from build123d import *

# Parameters (mm, degrees)
SKETCH_1_W          = 33
SKETCH_1_H          = 45
EXTRUDE_1_DEPTH     = 17
SKETCH_2_W          = 5
SKETCH_2_H          = 6
CUT_EXTRUDE_1_DEPTH = 44.407948581
SKETCH_4_R          = 3
EXTRUDE_2_DEPTH     = 6


with BuildPart() as part:
    # Эскиз1 → Бобышка-Вытянуть1 (new body)
    with BuildSketch(Plane.XY):
        Rectangle(SKETCH_1_W, SKETCH_1_H)
    extrude(amount=EXTRUDE_1_DEPTH)

    # Эскиз2 → Вырез-Вытянуть1 (cut, through all)
    with BuildSketch(Plane.ZY.offset(16.5)):
        Polygon((8, 3), (8, 10), (0, 10), (0, -10), (8, -10), (8, -3), align=None)
        with Locations((10.5, 0)):
            Rectangle(SKETCH_2_W, SKETCH_2_H)
    extrude(amount=-CUT_EXTRUDE_1_DEPTH, mode=Mode.SUBTRACT)

    # Эскиз4 → Бобышка-Вытянуть2 (add)
    with BuildSketch(Plane.XZ.offset(22.5)):
        with BuildLine():
            Line((-10, 17), (10, 17))
            ThreePointArc((10, 17), (0, 27), (-10, 17))
        make_face()
        with Locations((0, 21)):
            Circle(SKETCH_4_R, mode=Mode.SUBTRACT)
    extrude_2 = extrude(amount=-EXTRUDE_2_DEPTH)

    # Зеркальное отражение1: Бобышка-Вытянуть2 across plane
    add(extrude_2.mirror(Plane.ZX))


solid = part.part
Could you check a few things on this model? Use its own coordinates, in mm. A direction names the side the tool comes from. Give positions to 0.01 mm unless a question says otherwise; leave off trailing zeros. Order: outer loops, then holes, each group sorted by start corner. A loop starts at its lowest first (then second) coordinate and runs counter-clockwise, first axis right, second up.
1. Suppose I cut it at D-D (y = -12). Write out the boundary of the cut face in (x, z), plus the area to 3 significant figures.
Answers below:
outline: (-16.5, 0) - (16.5, 0) - (16.5, 17) - (-16.5, 17) - close
area: 561 mm2
2. For pin 1 (1.5 mm diameter, centred on x = 0.5, y = 2, fed in from -Z); pin 2 (5 mm diameter, centred on x = 12.5, y = 14, fed in from +Z); pin 3 (3.5 mm diameter, centred on x = 6, y = -5, fed in from -Z), each with a flat end and sliding along its axis, tell me the tip position at first contact or that it passes through.
Answers below:
pin 1: stops at z = 13
pin 2: stops at z = 17
pin 3: stops at z = 8
3. Suppose I cut it at C-C (z = 21). Write out the boundary of the cut face in (x, y), plus the area to 3 significant figures.
Answers below:
outline: (-9.17, -22.5) - (-3, -22.5) - (-3, -16.5) - (-9.17, -16.5) - close; (-9.17, 16.5) - (-3, 16.5) - (-3, 22.5) - (-9.17, 22.5) - close; (3, -22.5) - (9.17, -22.5) - (9.17, -16.5) - (3, -16.5) - close; (3, 16.5) - (9.17, 16.5) - (9.17, 22.5) - (3, 22.5) - close
area: 148 mm2
4. I need wall thicknesses on L1, parallel to Y at x = 3.5, z = 23.25; L2, parallel to Y at x = -3, z = 4.5; L3, parallel to Z at x = 0, y = 21.2. Which ranges of each line are inside material? Lowest first, please.
Answers below:
L1: y = -22.5 to -16.5, 16.5 to 22.5
L2: y = -22.5 to -10, 10 to 22.5
L3: z = 0 to 18, 24 to 27
5. Thinking about a two-plate mould opening in Z: for faces 1 (the cylindrical face through (-0.65, 19.54, 18.07)), 2 (the flat face through (0, -16, 0)), 3 (the flat face through (0, 3, 10)), which applies, +Z half, -Z half, draft (parallel to the pull), parting line (faces both ways), or undercut?
Answers below:
face 1: undercut
face 2: -Z half
face 3: draft
6. Which directions (+Z, -Z, +X, -X, +Y, -Y) give clear straight access to the entire face, cutting with the end or side of a thin tool? Please do faces 4 (the flat face through (0, -10, 4)), 5 (the cylindrical face through (0, -20, 27)), 6 (the flat face through (-2.4, -16.5, 23.2)).
Answers below:
face 4: -Z, +X, -X
face 5: +Z, +Y, -Y
face 6: +Z, +X, -X
7. Suppose I cut it at A-A (z = 12.5). Write out the boundary of the cut face in (x, y), plus the area to 3 significant figures.
Answers below:
outline: (-16.5, -22.5) - (16.5, -22.5) - (16.5, -3) - (-16.5, -3) - close; (-16.5, 3) - (16.5, 3) - (16.5, 22.5) - (-16.5, 22.5) - close
area: 1,290 mm2
8. Suppose I cut it at B-B (x = 0). Write out the boundary of the cut face in (y, z), plus the area to 3 significant figures.
Answers below:
outline: (-22.5, 0) - (-10, 0) - (-10, 8) - (-3, 8) - (-3, 13) - (3, 13) - (3, 8) - (10, 8) - (10, 0) - (22.5, 0) - (22.5, 18) - (16.5, 18) - (16.5, 17) - (-16.5, 17) - (-16.5, 18) - (-22.5, 18) - close; (-22.5, 24) - (-16.5, 24) - (-16.5, 27) - (-22.5, 27) - close; (16.5, 24) - (22.5, 24) - (22.5, 27) - (16.5, 27) - close
area: 623 mm2
